Verification items for the finished model (mm, model axes). A direction names the side the tool comes from. Round coordinates to 2 decimals unless told otherwise and drop trailing zeros. Write each loop counter-clockwise with the first axis right and the second up, starting at its lowest first coordinate (ties: lowest second). Pieces come first, ordered by that corner, then holes. Notation, with made-up numbers: (85.5, 88.25) - (108.5, 88.25) arc R21 cw to (108.5, 111.25) - close; hole circle Ø9 at (17.5, 78.25). An arc over 180 degrees is marked (long way). Write each question's results on one line, items separated by ' | '.
Autodesk Inventor part; units mm, degrees
ref_plane "Work Plane1" through (0, 40, 0) normal (0, 1, 0) x (-1, 0, 0)
ref_plane "Work Plane3" through (25, 40, 22.5) normal (-0.1736, 0.9848, 0) x (0, 0, -1)
ref_plane "YZ Plane" through (0, 0, 0) normal (1, 0, 0) x (0, 1, 0)
sketch "Sketch1" plane through (0, 0, 0) normal (1, 0, 0) x (0, 1, 0)
  circle A0 centre (0, 0) radius 19.5
  circle A1 centre (0, 0) radius 22.5
  dimension "d0" = 39
  dimension "d1" = 45
extrude "Extrusion1" add sketch "Sketch1" along normal mid plane 94
ref_plane "Work Plane1" through (0, 40, 0) normal (0, 1, 0) x (-1, 0, 0)
sketch "Sketch2" plane through (0, 40, 0) normal (0, 1, 0) x (-1, 0, 0)
  circle A0 centre (32, 0) radius 12.5
  circle A1 centre (32, 0) radius 7.9
  line L0 (47, -22.5) -> (47, 22.5)
  point P0 (0, 0)
  dimension "d6" = 25
  dimension "d7" = 15.8
  dimension "d19" = 15
extrude "Extrusion2" add sketch "Sketch2" against normal up to surface
sketch "Sketch3" plane through (0, 40, 0) normal (0, 1, 0) x (-1, 0, 0)
  line L0 (47, 22.5) -> (-47, 22.5)
  line L1 (-25, 22.5) -> (-25, -21.8926)
  line L2 (47, 22.5) -> (-47, 22.5)
  point P0 (0, 0)
  dimension "d16" = 25
ref_plane "Work Plane3" through (25, 40, 22.5) normal (-0.1736, 0.9848, 0) x (0, 0, -1)
sketch "Sketch4" plane through (25, 40, 22.5) normal (-0.1736, 0.9848, 0) x (0, 0, -1)
  ellipse E0 centre (22.5, 56.134) end of major axis (14.6, 56.134) minor radius 7.78
  circle A0 centre (22.5, -2.866) radius 7.9
  circle A1 centre (22.5, -2.866) radius 12.5
  ellipse E1 centre (22.5, 56.134) end of major axis (10, 56.134) minor radius 12.3101
  point P0 (22.5, 31.5661)
  dimension "d11" = 59
  dimension "d12" = 15.8
  dimension "d13" = 25
extrude "Extrusion3" add sketch "Sketch4" against normal up to surface contours A1
mirror "Mirror1" about plane through (0, 0, 0) normal (0, 1, 0) of "Extrusion2", "Extrusion3"
properties part number "JuntaRodilla" material "PLA"
(1) Thickness scan on L1, parallel to Z at x = 29.5, y = -33; L2, parallel to Z at x = -36.5, y = 0; L3, parallel to X at y = 31, z = 0. Record the ranges inside material, lowest first.
Answer:
L1: -12.5 to -7.89, 7.89 to 12.5 | L2: -22.5 to -19.5, 19.5 to 22.5 | L3: -44.5 to -39.9, -24.1 to -19.5, 16.8 to 21.48, 37.52 to 42.19
(2) Mould release check, pull along Y, two halves, no side actions. Record for faces 6 (the cylindrical face through (-43.923, 29.503, 3.755)), 7 (the flat face through (35.857, 41.914, 0.175)), 8 (the flat face through (35.857, -41.914, -0.175)), 9 (the cylindrical face through (36.099, -31.917, -4.247)): released by +Y, released by -Y, zero draft, split by the parting line, or undercut.
Answer:
face 6: zero draft | face 7: released by +Y | face 8: released by -Y | face 9: undercut
(3) Section check D-D (x = -2). Record the cut outline in (y, z), plus the area to 3 significant figures.
Answer:
outline: circle Ø45 at (0, 0); hole circle Ø39 at (0, 0) | area: 396 mm2
(4) Section check B-B (z = 9.5). Record the cut outline in (x, y), plus the area to 3 significant figures.
Answer:
outline: (-47, -20.4) - (-40.12, -20.4) - (-40.12, -40) - (-23.88, -40) - (-23.88, -20.4) - (23.12, -20.4) - (19.82, -39.09) - (35.82, -41.91) - (39.62, -20.4) - (47, -20.4) - (47, -17.03) - (-47, -17.03) - close; (-47, 17.03) - (47, 17.03) - (47, 20.4) - (39.62, 20.4) - (35.82, 41.91) - (19.82, 39.09) - (23.12, 20.4) - (-23.88, 20.4) - (-23.88, 40) - (-40.12, 40) - (-40.12, 20.4) - (-47, 20.4) - close | area: 1,930 mm2
(5) Section check A-A (y = 0). Record the cut outline in (x, z).
Answer:
outline: (-47, -22.5) - (47, -22.5) - (47, -19.5) - (-47, -19.5) - close; (-47, 19.5) - (47, 19.5) - (47, 22.5) - (-47, 22.5) - close
(6) Set-up check for faces 1 (the cylindrical face through (30.9, -22.5, -0.1)), 2 (the cylindrical face through (-43.923, -29.503, -3.755)), 3 (the flat face through (-40.2, 40, 0.2)), 4 (the flat face through (-32.2, -40, -8.2)), 5 (the flat face through (47, -17, 10)): record each of +Z, -Z, +X, -X, +Y, -Y from which the full face is reachable in a straight line by a thin tool's end or side.
Answer:
face 1: none | face 2: -Y | face 3: +Z, -Z, -X, +Y | face 4: +Z, -Z, -X, -Y | face 5: +Z, -Z, +X, +Y, -Y
(7) Go/stop test with flat-tipped pins: pin 1 Ø2 at (x, y) = (-29.5, 6) entering from -Z; pin 2 Ø12 at (x, z) = (-14.5, 14.5) entering from -Y; pin 3 Ø12.5 at (x, z) = (-32, 0) entering from -Y. Record where each tip stops, or that it passes through.
Answer:
pin 1: z = -21.94 | pin 2: y = -20.83 | pin 3: y = -22.5
(8) Section check C-C (x = -32). Record the cut outline in (y, z).
Answer:
outline: (-40, -12.5) - (-18.71, -12.5) arc R22.5 ccw to (18.71, -12.5) - (40, -12.5) - (40, -7.9) - (21.07, -7.9) arc R22.5 ccw to (21.07, 7.9) - (40, 7.9) - (40, 12.5) - (18.71, 12.5) arc R22.5 ccw to (-18.71, 12.5) - (-40, 12.5) - (-40, 7.9) - (-21.07, 7.9) arc R22.5 ccw to (-21.07, -7.9) - (-40, -7.9) - close; hole circle Ø39 at (0, 0)
